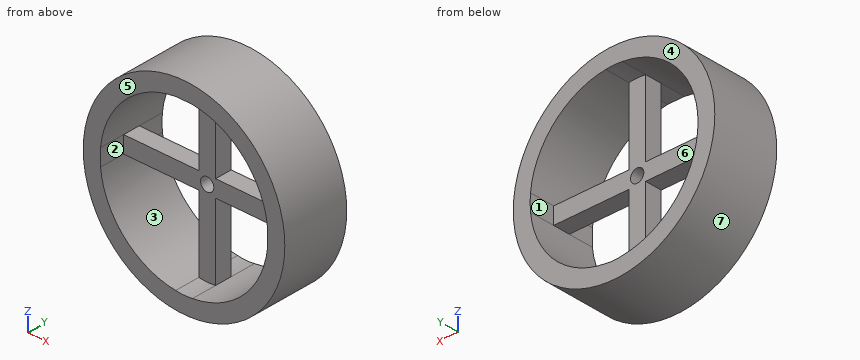
from build123d import *

# Parameters (mm, degrees)
F0_R     = 76.2
F0_R_2   = 5
F1_DEPTH = 25.4
F2_R     = 5
F3_DEPTH = 19
F4_R     = 5
F5_DEPTH = 19


with BuildPart() as f1:
    # F0 (on Front) → F1 (new body, symmetric)
    with BuildSketch(Plane.XZ):
        Circle(F0_R)
        with BuildLine():
            ThreePointArc((-6.35, -63.181702), (-44.901281, -44.901281), (-63.181702, -6.35))
            Line((-63.181702, -6.35), (-6.35, -6.35))
            Line((-6.35, -6.35), (-6.35, -63.181702))
        make_face(mode=Mode.SUBTRACT)
        with BuildLine():
            Line((6.35, -6.35), (63.181702, -6.35))
            ThreePointArc((63.181702, -6.35), (44.901281, -44.901281), (6.35, -63.181702))
            Line((6.35, -63.181702), (6.35, -6.35))
        make_face(mode=Mode.SUBTRACT)
        with BuildLine():
            ThreePointArc((-63.181702, 6.35), (-44.901281, 44.901281), (-6.35, 63.181702))
            Line((-6.35, 63.181702), (-6.35, 6.35))
            Line((-6.35, 6.35), (-63.181702, 6.35))
        make_face(mode=Mode.SUBTRACT)
        Circle(F0_R_2, mode=Mode.SUBTRACT)
        with BuildLine():
            Line((6.35, 6.35), (6.35, 63.181702))
            ThreePointArc((6.35, 63.181702), (44.901281, 44.901281), (63.181702, 6.35))
            Line((63.181702, 6.35), (6.35, 6.35))
        make_face(mode=Mode.SUBTRACT)
    extrude(amount=F1_DEPTH, both=True)

    # F2 (on face) → F3 (cut)
    with BuildSketch(Plane.XZ.offset(25.4)):
        with BuildLine():
            Line((-6.35, 6.35), (-63.181702, 6.35))
            ThreePointArc((-63.181702, 6.35), (-63.322942, 0), (-63.181702, -6.35))
            Line((-63.181702, -6.35), (-6.35, -6.35))
            Line((-6.35, -6.35), (-6.35, -63.181702))
            ThreePointArc((-6.35, -63.181702), (0, -63.649263), (6.35, -63.181702))
            Line((6.35, -63.181702), (6.35, -6.35))
            Line((6.35, -6.35), (63.181702, -6.35))
            ThreePointArc((63.181702, -6.35), (63.272965, 0), (63.181702, 6.35))
            Line((63.181702, 6.35), (6.35, 6.35))
            Line((6.35, 6.35), (6.35, 63.181702))
            ThreePointArc((6.35, 63.181702), (0, 63.211711), (-6.35, 63.181702))
            Line((-6.35, 63.181702), (-6.35, 6.35))
        make_face()
        Circle(F2_R, mode=Mode.SUBTRACT)
    extrude(amount=-F3_DEPTH, mode=Mode.SUBTRACT)

    # F4 (on face) → F5 (cut)
    with BuildSketch(Plane(origin=(0, 25.4, 0), x_dir=(-1, 0, 0), z_dir=(0, 1, 0))):
        with BuildLine():
            Line((6.35, 6.35), (6.35, 63.181702))
            ThreePointArc((6.35, 63.181702), (0, 63.522837), (-6.35, 63.181702))
            Line((-6.35, 63.181702), (-6.35, 6.35))
            Line((-6.35, 6.35), (-63.181702, 6.35))
            ThreePointArc((-63.181702, 6.35), (-63.393876, 0), (-63.181702, -6.35))
            Line((-63.181702, -6.35), (-6.35, -6.35))
            Line((-6.35, -6.35), (-6.35, -63.181702))
            ThreePointArc((-6.35, -63.181702), (0, -63.739805), (6.35, -63.181702))
            Line((6.35, -63.181702), (6.35, -6.35))
            Line((6.35, -6.35), (63.181702, -6.35))
            ThreePointArc((63.181702, -6.35), (63.425239, 0), (63.181702, 6.35))
            Line((63.181702, 6.35), (6.35, 6.35))
        make_face()
        Circle(F4_R, mode=Mode.SUBTRACT)
    extrude(amount=-F5_DEPTH, mode=Mode.SUBTRACT)


solid = f1.part
Geometry check sheet. Reference: the model listing, model coordinates, mm. Face numbers are marked on the shaded views. A direction names the side the tool comes from. Round coordinates to 2 decimals unless told otherwise and drop trailing zeros. Loops run counter-clockwise (first coordinate to the right, second up) from the corner with the lowest first, then second, coordinate; pieces in that order, holes last.
Item 1: Cross-section at A-A on x = 0. Record the boundary of the cut face in (y, z).
Item 2: Access from +Z, -Z, +X, -X, +Y, -Y to the whole of each face (thin tool, end or side, straight path). Record for the marked faces 1, 2, 3 and 4.
Item 3: Thickness scan on line 1 (Z direction, x = 0, y = 1); line 2 (X direction, y = 1, z = 25); line 3 (Z direction, x = -39.5, y = -1). Record the ranges inside material, lowest first.
Item 4: Cross-section at C-C on y = -19. Record the boundary of the cut face in (x, z), then the cut area to 3 significant figures.
Item 5: Cross-section at B-B on z = 0. Record the boundary of the cut face in (x, y).
Item 6: Gauge pin test, flat ends, axial feed: pin 1 (12 mm diameter, centred on y = -5, z = -15.5, fed in from -X); pin 2 (4 mm diameter, centred on y = -14, z = -3, fed in from +X); pin 3 (4 mm diameter, centred on x = 29, y = 2, fed in from +Z). Record the tip position at first contact, or that the pin passes through.
Item 7: Mould release check, pull along X, two halves, no side actions. Record for the marked faces 5, 6 and 7: pulls with the +X half, pulls with the -X half, needs draft (parallel to the pull), parting line crosses it, or undercut.
Item 8: Cross-section at D-D on z = 48.5. Record the boundary of the cut face in (x, y).
Answer sheet:
1. outline: (-25.4, -76.2) - (25.4, -76.2) - (25.4, -63.74) - (6.4, -63.74) - (6.4, -5) - (-6.4, -5) - (-6.4, -63.65) - (-25.4, -63.65) - close; (-25.4, 63.21) - (-6.4, 63.21) - (-6.4, 5) - (6.4, 5) - (6.4, 63.52) - (25.4, 63.52) - (25.4, 76.2) - (-25.4, 76.2) - close
2. face 1: +Y
2. face 2: -Y
2. face 3: +Y, -Y
2. face 4: +Z, -Z, +X, -X, +Y
3. line 1: z = -76.2 to -5, 5 to 76.2
3. line 2: x = -71.98 to -58.37, -6.35 to 6.35, 58.37 to 71.98
3. line 3: z = -65.16 to -49.72, -6.35 to 6.35, 49.72 to 65.16
4. outline: circle Ø152.4 at (0, 0); hole (-63.18, -6.35) arc R63.5 ccw to (-6.35, -63.18) arc R43.35 ccw to (6.35, -63.18) arc R63.5 ccw to (63.18, -6.35) arc R220.96 ccw to (63.18, 6.35) arc R63.5 ccw to (6.35, 63.18) arc R671.86 ccw to (-6.35, 63.18) arc R63.5 ccw to (-63.18, 6.35) arc R142.82 ccw to start
4. area: 5,580 mm2
5. outline: (-76.2, -25.4) - (-63.32, -25.4) - (-63.32, -6.4) - (-5, -6.4) - (-5, 6.4) - (-63.43, 6.4) - (-63.43, 25.4) - (-76.2, 25.4) - close; (5, -6.4) - (63.27, -6.4) - (63.27, -25.4) - (76.2, -25.4) - (76.2, 25.4) - (63.39, 25.4) - (63.39, 6.4) - (5, 6.4) - close
6. pin 1: stops at x = -75.61
6. pin 2: stops at x = 76.19
6. pin 3: stops at z = 71.26
7. face 5: needs draft
7. face 6: undercut
7. face 7: parting line crosses it
8. outline: (-58.77, -25.4) - (-40.99, -25.4) - (-40.99, 25.4) - (-58.77, 25.4) - close; (-6.35, -6.4) - (6.35, -6.4) - (6.35, 6.4) - (-6.35, 6.4) - close; (40.99, -25.4) - (58.77, -25.4) - (58.77, 25.4) - (40.99, 25.4) - close
